Design review of the part shown in the three views and the two pictorial views. Dimensions are in mm from the part's minimum x, y and z. A direction names the side the tool comes from. Round coordinates to 2 decimals unless told otherwise and drop trailing zeros. Loops run counter-clockwise (first coordinate to the right, second up) from the corner with the lowest first, then second, coordinate; pieces in that order, holes last. Notation, with made-up numbers: (38.5, 82) - (48.5, 82) arc R30 ccw to (48.5, 116) - close; hole circle Ø8 at (58.5, 0). An arc over 180 degrees is marked (long way). Return JSON: item names as keys, results as strings. Group by question number.
(1) Clearance check with flat-ended pins moving along their axes: pin 1 (10 mm diameter, centred on x = 17.5, y = 4, fed in from +Z); pin 2 (4.5 mm diameter, centred on y = 4.25, z = 13, fed in from +X); pin 3 (10 mm diameter, centred on y = 3, z = 15.5, fed in from +X). State where each tip first meets the part, or that it passes through.
(2) We need section A-A, the plane y = 14.25. Write out the cut boundary in (x, z).
(3) The part is to be moulded in two halves that separate along X. For the marked faces 3, 4 and 5, say which applies: pulls with the +X half, pulls with the -X half, needs draft (parallel to the pull), parting line crosses it, or undercut.
(4) Wall thickness on L1, parallel to Y at x = 2.05, z = 13; L2, parallel to Y at x = 12, z = 2; L3, parallel to X at y = 9.75, z = 1: over which ranges is each line inside the solid? List them lowest first. Write a range as [from, to].
(5) We need section B-B, the plane z = 13. Write out the cut boundary in (x, y).
(6) For the marked faces 1 and 2, list the 3-axis set-ups (+Z, -Z, +X, -X, +Y, -Y) from which the entire face can be reached by the end or side of a thin tool; tool diameter is ignored.
(7) We need section C-C, the plane x = 12. Write out the cut boundary in (y, z), and give its area (3 significant figures).
(8) We need section D-D, the plane y = 9.25. Write out the cut boundary in (x, z), and give its area (3 significant figures).
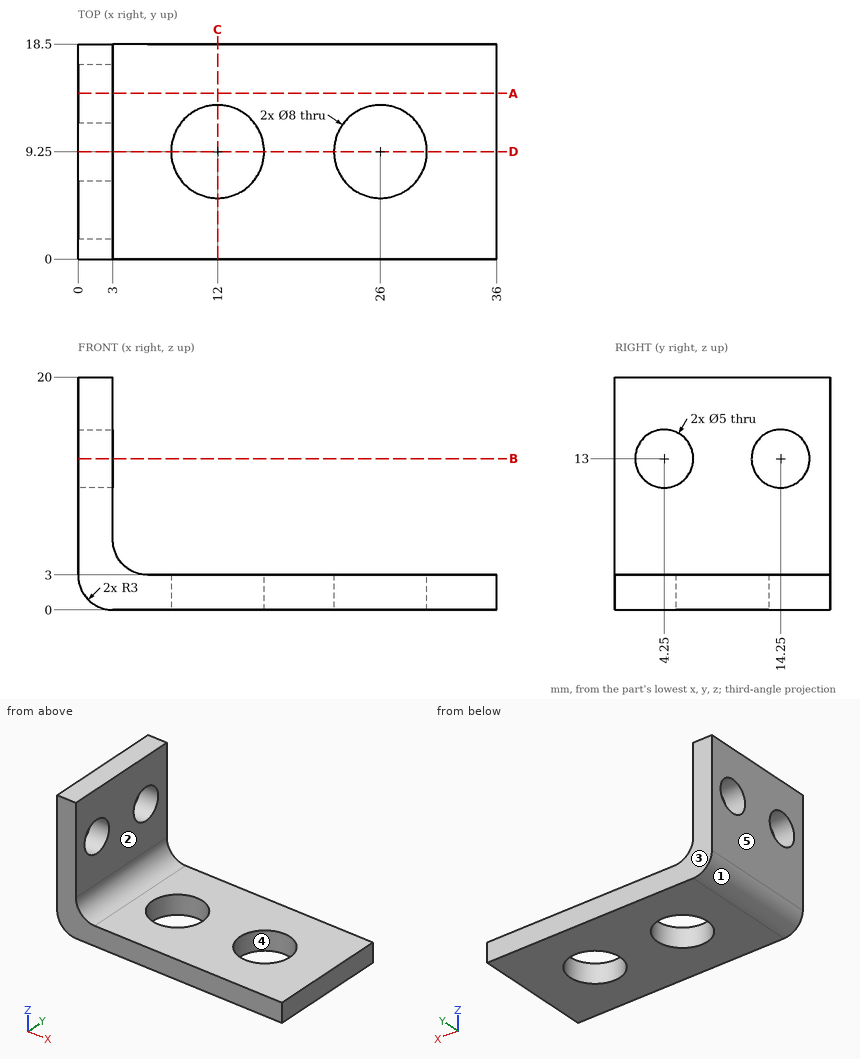
Solutions:
{
 "1": {"pin 1": "z = 3", "pin 2": "through", "pin 3": "x = 3"},
 "2": {"outline": "(0, 3) arc R3 ccw to (3, 0) - (36, 0) - (36, 3) - (6, 3) arc R3 cw to (3, 6) - (3, 10.5) - (0, 10.5) - close; (0, 15.5) - (3, 15.5) - (3, 20) - (0, 20) - close"},
 "3": {"face 3": "needs draft", "face 4": "undercut", "face 5": "pulls with the -X half"},
 "4": {"L1": "[0, 1.75], [6.75, 11.75], [16.75, 18.5]", "L2": "[0, 5.25], [13.25, 18.5]", "L3": "[0.76, 8.03], [15.97, 22.03], [29.97, 36]"},
 "5": {"outline": "(0, 0) - (3, 0) - (3, 1.75) - (0, 1.75) - close; (0, 6.75) - (3, 6.75) - (3, 11.75) - (0, 11.75) - close; (0, 16.75) - (3, 16.75) - (3, 18.5) - (0, 18.5) - close"},
 "6": {"face 1": "-Z, -X, +Y, -Y", "face 2": "+Z, +X, +Y, -Y"},
 "7": {"outline": "(0, 0) - (5.25, 0) - (5.25, 3) - (0, 3) - close; (13.25, 0) - (18.5, 0) - (18.5, 3) - (13.25, 3) - close", "area": "31.5 mm^2"},
 "8": {"outline": "(0, 3) arc R3 ccw to (3, 0) - (8, 0) - (8, 3) - (6, 3) arc R3 cw to (3, 6) - (3, 20) - (0, 20) - close; (16, 0) - (22, 0) - (22, 3) - (16, 3) - close; (30, 0) - (36, 0) - (36, 3) - (30, 3) - close", "area": "111 mm^2"}
}
